from build123d import *

# Parameters (mm, degrees)
RESSALTO_EXTRUS_O1_DEPTH   = 22
ESBO_O2_W                  = 7
ESBO_O2_H                  = 13.5
CORTE_EXTRUS_O1_DEPTH      = 23
CORTE_EXTRUS_O2_DEPTH      = 10
CORTE_EXTRUS_O2_DEPTH_BACK = 35


with BuildPart() as part:
    # Esboço1 → Ressalto-extrusão1 (new body)
    with BuildSketch(Plane.XY):
        with BuildLine():
            Line((7.5, 6.614378278), (7.5, 30))
            Line((7.5, 30), (-7.5, 30))
            Line((-7.5, 30), (-7.5, 15))
            ThreePointArc((-7.5, 15), (-8.964466094, 11.464466094), (-12.5, 10))
            Line((-12.5, 10), (-25, 10))
            ThreePointArc((-25, 10), (-35, 0), (-25, -10))
            Line((-25, -10), (0, -10))
            ThreePointArc((0, -10), (9.114378278, -4.114378278), (7.5, 6.614378278))
        make_face()
        with BuildLine():
            Line((-25, 4.5), (0, 4.5))
            ThreePointArc((0, 4.5), (4.5, 0), (0, -4.5))
            Line((0, -4.5), (-25, -4.5))
            ThreePointArc((-25, -4.5), (-29.5, 0), (-25, 4.5))
        make_face(mode=Mode.SUBTRACT)
    extrude(amount=RESSALTO_EXTRUS_O1_DEPTH)

    # Esboço2 → Corte-extrusão1 (cut)
    with BuildSketch(Plane(origin=(0, 30, 0), x_dir=(1, 0, 0), z_dir=(0, 1, 0))):
        with Locations((0, -11)):
            Rectangle(ESBO_O2_W, ESBO_O2_H)
    extrude(amount=-CORTE_EXTRUS_O1_DEPTH, mode=Mode.SUBTRACT)

    # Esboço3 → Corte-extrusão2 (cut, two sides)
    with BuildSketch(Plane(origin=(7.5, 0, 0), x_dir=(0, 0, -1), z_dir=(1, 0, 0))) as corte_extrus_o2_sk:
        with BuildLine():
            Line((-15.5, 15.807189139), (-15.5, 20.807189139))
            ThreePointArc((-15.5, 20.807189139), (-11, 25.307189139), (-6.5, 20.807189139))
            Line((-6.5, 20.807189139), (-6.5, 15.807189139))
            ThreePointArc((-6.5, 15.807189139), (-11, 11.307189139), (-15.5, 15.807189139))
        make_face()
    extrude(amount=CORTE_EXTRUS_O2_DEPTH, mode=Mode.SUBTRACT)
    extrude(corte_extrus_o2_sk.sketch, amount=-CORTE_EXTRUS_O2_DEPTH_BACK, mode=Mode.SUBTRACT)


solid = part.part
Could you check a few things on this model? Use its own coordinates, in mm. A direction names the side the tool comes from. Give positions to 0.01 mm unless a question says otherwise; leave off trailing zeros. Order: outer loops, then holes, each group sorted by start corner. A loop starts at its lowest first (then second) coordinate and runs counter-clockwise, first axis right, second up.
1. Suppose I cut it at A-A (x = -20). Write out the boundary of the cut face in (y, z), plus the area to 3 significant figures.
Answers below:
outline: (-10, 0) - (-4.5, 0) - (-4.5, 22) - (-10, 22) - close; (4.5, 0) - (10, 0) - (10, 22) - (4.5, 22) - close
area: 242 mm2
2. Suppose I cut it at D-D (z = 17). Write out the boundary of the cut face in (x, y).
Answers below:
outline: (-25, -10) - (0, -10) arc R10 ccw to (7.5, 6.61) - (7.5, 30) - (3.5, 30) - (3.5, 7) - (-3.5, 7) - (-3.5, 30) - (-7.5, 30) - (-7.5, 15) arc R5 cw to (-12.5, 10) - (-25, 10) arc R10 ccw to start; hole (-25, -4.5) - (0, -4.5) arc R4.5 ccw to (0, 4.5) - (-25, 4.5) arc R4.5 ccw to start
3. For pin 1 (11 mm diameter, centred on x = -17.5, z = 6.5, fed in from +Y); pin 2 (7 mm diameter, centred on y = 15, z = 13, fed in from +X); pin 3 (12 mm diameter, centred on y = 22.5, z = 14, fed in from -X); pin 4 (1.5 mm diameter, centred on x = -9, y = 17.5, fed in from -Z), each with a flat end and sliding along its axis, tell me the tip position at first contact or that it passes through.
Answers below:
pin 1: stops at y = 10.03
pin 2: stops at x = 7.5
pin 3: stops at x = -7.5
pin 4: passes through
4. Suppose I cut it at B-B (y = 18.5). Write out the boundary of the cut face in (x, z), plus the area to 4 significant figures.
Answers below:
outline: (-7.5, 0) - (7.5, 0) - (7.5, 6.5) - (3.5, 6.5) - (3.5, 4.25) - (-3.5, 4.25) - (-3.5, 6.5) - (-7.5, 6.5) - close; (-7.5, 15.5) - (-3.5, 15.5) - (-3.5, 17.75) - (3.5, 17.75) - (3.5, 15.5) - (7.5, 15.5) - (7.5, 22) - (-7.5, 22) - close
area: 163.5 mm2
5. Thinking about a two-plate mould opening in X: for faces 6 (the cylindrical face through (9.047, -4.26, 10.846)), 7 (the flat face through (0, 19, 4.25)), 8 (the flat face through (-5, 18, 15.5)), which applies, +X half, -X half, draft (parallel to the pull), parting line (faces both ways), or undercut?
Answers below:
face 6: +X half
face 7: undercut
face 8: draft
6. I need wall thicknesses on L1, parallel to Y at x = -12.5, z = 17.25; L2, parallel to Y at x = -2.5, z = 14.5; L3, parallel to X at y = 0, z = 10.5. Which ranges of each line are inside material? Lowest first, please.
Answers below:
L1: y = -10 to -4.5, 4.5 to 10
L2: y = -10 to -4.5, 4.5 to 7
L3: x = -35 to -29.5, 4.5 to 10
7. Which directions (+Z, -Z, +X, -X, +Y, -Y) give clear straight access to the entire face, cutting with the end or side of a thin tool? Please do faces 1 (the flat face through (-19, 10, 11)), 2 (the cylindrical face through (-5.65, 11.31, 10.9)), 3 (the cylindrical face through (4.5, 0.1, 10.8)), 4 (the flat face through (3.5, 19, 16)), 5 (the flat face through (-8, 10, 0)).
Answers below:
face 1: +Z, -Z, -X, +Y
face 2: +X, -X
face 3: +Z, -Z
face 4: +Y
face 5: -Z, +X, -X, +Y, -Y
8. Suppose I cut it at C-C (z = 11). Write out the boundary of the cut face in (x, y), plus the area to 3 significant figures.
Answers below:
outline: (-25, -10) - (0, -10) arc R10 ccw to (7.5, 6.61) - (7.5, 11.31) - (3.5, 11.31) - (3.5, 7) - (-3.5, 7) - (-3.5, 11.31) - (-9.13, 11.31) arc R5 cw to (-12.5, 10) - (-25, 10) arc R10 ccw to start; (-7.5, 25.31) - (-3.5, 25.31) - (-3.5, 30) - (-7.5, 30) - close; (3.5, 25.31) - (7.5, 25.31) - (7.5, 30) - (3.5, 30) - close; hole (-25, -4.5) - (0, -4.5) arc R4.5 ccw to (0, 4.5) - (-25, 4.5) arc R4.5 ccw to start
area: 564 mm2
